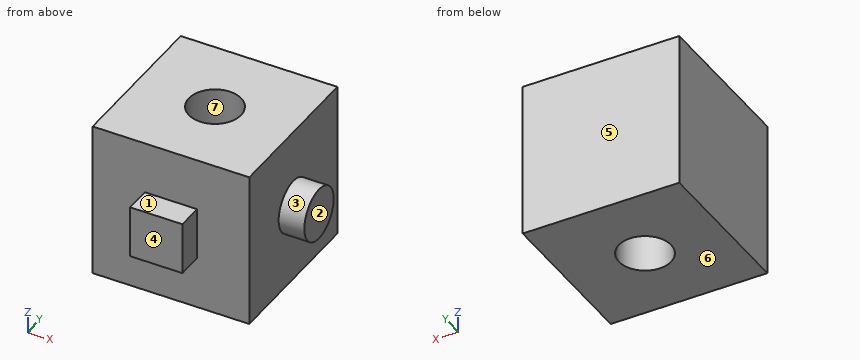
```python
from build123d import *

# Parameters (mm, degrees)
F0_W     = 76.2
F0_H     = 76.2
F1_DEPTH = 76.2
F2_R     = 12.7
F3_DEPTH = 58.42
F5_D     = 25.4
F6_W     = 25.4
F6_H     = 25.4
F7_DEPTH = 12.7


with BuildPart() as f1:
    # F0 (on Front) → F1 (new body)
    with BuildSketch(Plane.XZ):
        with Locations((7.805411, 12.657838)):
            Rectangle(F0_W, F0_H)
    extrude(amount=F1_DEPTH)

    # F2 (on Right) → F3 (join)
    with BuildSketch(Plane.YZ):
        with Locations((-38.1, 12.657838)):
            Circle(F2_R)
    extrude(amount=F3_DEPTH)

    # F5 (through all)
    with Locations(Plane.XY.offset(50.757838)):
        with Locations((7.805411, -38.1)):
            Hole(F5_D / 2)

    # F6 (on face) → F7 (join)
    with BuildSketch(Plane.XZ.offset(76.2)):
        with Locations((7.805411, 12.7)):
            Rectangle(F6_W, F6_H)
    extrude(amount=F7_DEPTH)


solid = f1.part
```
Build history of the part. All positions in model axes, mm. Face numbers are marked on the shaded views. A direction names the side the tool comes from. Round coordinates to 2 decimals unless told otherwise and drop trailing zeros. Order: outer loops, then holes, each group sorted by start corner. A loop starts at its lowest first (then second) coordinate and runs counter-clockwise, first axis right, second up. Notation, with made-up numbers: (79.5, 61) -> (122.5, 61) arc R20 cw to (122.5, 87) -> close; hole circle Ø9 at (79, 60.25). An arc over 180 degrees is marked (long way). Answer in a Markdown table with one row per item.
1) Band-saw the part on D-D on y = -20. Give the cut face in (x, z).
Values:
| item | result |
|---|---|
| outline | (-30.29, -25.44) -> (45.91, -25.44) -> (45.91, 50.76) -> (-30.29, 50.76) -> close |
2) Band-saw the part on A-A on y = -38.1. Give the cut face in (x, z).
Values:
| item | result |
|---|---|
| outline | (-30.29, -25.44) -> (-4.89, -25.44) -> (-4.89, 50.76) -> (-30.29, 50.76) -> close; (20.51, -25.44) -> (45.91, -25.44) -> (45.91, -0.04) -> (58.42, -0.04) -> (58.42, 25.36) -> (45.91, 25.36) -> (45.91, 50.76) -> (20.51, 50.76) -> close |
3) Band-saw the part on B-B on z = 27.5. Give the cut face in (x, y), and give its area (3 significant figures).
Values:
| item | result |
|---|---|
| outline | (-30.29, -76.2) -> (45.91, -76.2) -> (45.91, 0) -> (-30.29, 0) -> close; hole circle Ø25.4 at (7.81, -38.1) |
| area | 5,300 mm2 |
4) Pin check, flat tips, straight feed: P1, Ø10, axis at x = 12.5, y = -83.5, coming from the -Z side; P2, Ø6.5, axis at x = 14, y = -81.5, coming from the +Z side; P3, Ø6, axis at x = -6, z = -14.5, coming from the -Y side. Stop position of each tip, or through.
Values:
| item | result |
|---|---|
| P1 | z = 0 |
| P2 | z = 25.4 |
| P3 | y = -76.2 |
5) Mould opens along Y. For the marked faces 4, 5, 6 and 7 say: released by +Y, released by -Y, zero draft, split by the parting line, or undercut.
Values:
| item | result |
|---|---|
| face 4 | released by -Y |
| face 5 | released by +Y |
| face 6 | zero draft |
| face 7 | undercut |
6) Which spindle directions (+Z, -Z, +X, -X, +Y, -Y) get a long thin tool onto all of the face, cutting with end or side? Do the marked faces 1, 2 and 3. Say none if no direction does.
Values:
| item | result |
|---|---|
| face 1 | +Z, +X, -X, -Y |
| face 2 | +Z, -Z, +X, +Y, -Y |
| face 3 | +X |
7) Band-saw the part on C-C on x = 15. Give the cut face in (y, z).
Values:
| item | result |
|---|---|
| outline | (-88.9, 0) -> (-76.2, 0) -> (-76.2, -25.44) -> (-48.57, -25.44) -> (-48.57, 50.76) -> (-76.2, 50.76) -> (-76.2, 25.4) -> (-88.9, 25.4) -> close; (-27.63, -25.44) -> (0, -25.44) -> (0, 50.76) -> (-27.63, 50.76) -> close |
8) Wall check: L1, parallel to X at y = -38, z = 22; L2, parallel to X at y = -38, z = 33; L3, parallel to X at y = -79, z = 22.5. Give the ranges that are in metal, low to high.
Values:
| item | result |
|---|---|
| L1 | -30.29 to -4.89, 20.51 to 58.42 |
| L2 | -30.29 to -4.89, 20.51 to 45.91 |
| L3 | -4.89 to 20.51 |
